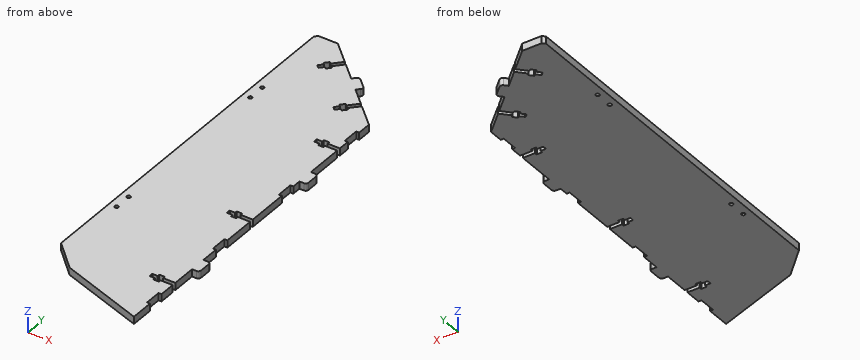
```python
from build123d import *

# Parameters (mm, degrees)
MODEL_R             = 1.6637
BOSS_EXTRUDE1_DEPTH = 6.6


with BuildPart() as part:
    # Model → Boss-Extrude1 (new body)
    with BuildSketch(Plane.XY):
        with BuildLine():
            Line((-2.7, 21.1), (0, 21.1))
            Line((0, 21.1), (0, 0))
            Line((0, 0), (-76.35, 26.1117))
            Line((-76.35, 26.1117), (-100, 49.2))
            Line((-100, 49.2), (-100, 380.9))
            Line((-100, 380.9), (-97.5, 383.4))
            Line((-97.5, 383.4), (-80, 383.4))
            Line((-80, 383.4), (-61.92031318, 366.450293606))
            Line((-61.92031318, 366.450293606), (-69.443665597, 358.42538436))
            Line((-69.443665597, 358.42538436), (-70.599982066, 359.50943105))
            ThreePointArc((-70.599982066, 359.50943105), (-70.958073277, 359.644402505), (-71.306721232, 359.486633012))
            Line((-71.306721232, 359.486633012), (-74.042485748, 356.568484196))
            ThreePointArc((-74.042485748, 356.568484196), (-74.177457203, 356.210392984), (-74.01968771, 355.861745029))
            Line((-74.01968771, 355.861745029), (-72.863371242, 354.77769834))
            Line((-72.863371242, 354.77769834), (-75.941106322, 351.494780921))
            ThreePointArc((-75.941106322, 351.494780921), (-76.076077777, 351.13668971), (-75.918308284, 350.788041755))
            Line((-75.918308284, 350.788041755), (-74.057988413, 349.043991876))
            ThreePointArc((-74.057988413, 349.043991876), (-73.699897202, 348.909020421), (-73.351249247, 349.066789913))
            Line((-73.351249247, 349.066789913), (-70.273514167, 352.349707332))
            Line((-70.273514167, 352.349707332), (-69.117197698, 351.265660643))
            ThreePointArc((-69.117197698, 351.265660643), (-68.759106487, 351.130689188), (-68.410458532, 351.288458681))
            Line((-68.410458532, 351.288458681), (-65.674694016, 354.206607497))
            ThreePointArc((-65.674694016, 354.206607497), (-65.539722561, 354.564698709), (-65.697492054, 354.913346664))
            Line((-65.697492054, 354.913346664), (-66.853808523, 355.997393353))
            Line((-66.853808523, 355.997393353), (-59.330456105, 364.022302598))
            Line((-59.330456105, 364.022302598), (-45.469249226, 351.02742115))
            Line((-45.469249226, 351.02742115), (-42.733484711, 353.945569966))
            ThreePointArc((-42.733484711, 353.945569966), (-40.990244935, 354.73441743), (-39.199788878, 354.059560154))
            Line((-39.199788878, 354.059560154), (-31.904416837, 347.220148866))
            ThreePointArc((-31.904416837, 347.220148866), (-31.115569373, 345.47690909), (-31.790426649, 343.686453033))
            Line((-31.790426649, 343.686453033), (-34.526191164, 340.768304216))
            Line((-34.526191164, 340.768304216), (-20.664984286, 327.773422768))
            Line((-20.664984286, 327.773422768), (-28.188336703, 319.748513522))
            Line((-28.188336703, 319.748513522), (-29.344653172, 320.832560211))
            ThreePointArc((-29.344653172, 320.832560211), (-29.702744383, 320.967531667), (-30.051392338, 320.809762174))
            Line((-30.051392338, 320.809762174), (-32.787156854, 317.891613357))
            ThreePointArc((-32.787156854, 317.891613357), (-32.922128309, 317.533522146), (-32.764358816, 317.184874191))
            Line((-32.764358816, 317.184874191), (-31.608042348, 316.100827502))
            Line((-31.608042348, 316.100827502), (-34.685777428, 312.817910083))
            ThreePointArc((-34.685777428, 312.817910083), (-34.820748883, 312.459818871), (-34.66297939, 312.111170916))
            Line((-34.66297939, 312.111170916), (-32.802659519, 310.367121038))
            ThreePointArc((-32.802659519, 310.367121038), (-32.444568308, 310.232149583), (-32.095920353, 310.389919075))
            Line((-32.095920353, 310.389919075), (-29.018185273, 313.672836494))
            Line((-29.018185273, 313.672836494), (-27.861868804, 312.588789805))
            ThreePointArc((-27.861868804, 312.588789805), (-27.503777593, 312.45381835), (-27.155129638, 312.611587842))
            Line((-27.155129638, 312.611587842), (-24.419365122, 315.529736659))
            ThreePointArc((-24.419365122, 315.529736659), (-24.284393667, 315.88782787), (-24.44216316, 316.236475825))
            Line((-24.44216316, 316.236475825), (-25.598479629, 317.320522515))
            Line((-25.598479629, 317.320522515), (-18.075127211, 325.34543176))
            Line((-18.075127211, 325.34543176), (0, 308.4))
            Line((0, 308.4), (0, 295.7))
            Line((0, 295.7), (-2.7, 295.7))
            Line((-2.7, 295.7), (-2.7, 280.7))
            Line((-2.7, 280.7), (0, 280.7))
            Line((0, 280.7), (0, 270.3))
            Line((0, 270.3), (-11, 270.3))
            Line((-11, 270.3), (-11, 271.885))
            ThreePointArc((-11, 271.885), (-11.146446609, 272.238553391), (-11.5, 272.385))
            Line((-11.5, 272.385), (-15.5, 272.385))
            ThreePointArc((-15.5, 272.385), (-15.853553391, 272.238553391), (-16, 271.885))
            Line((-16, 271.885), (-16, 270.3))
            Line((-16, 270.3), (-20.5, 270.3))
            ThreePointArc((-20.5, 270.3), (-20.853553391, 270.153553391), (-21, 269.8))
            Line((-21, 269.8), (-21, 267.25))
            ThreePointArc((-21, 267.25), (-20.853553391, 266.896446609), (-20.5, 266.75))
            Line((-20.5, 266.75), (-16, 266.75))
            Line((-16, 266.75), (-16, 265.165))
            ThreePointArc((-16, 265.165), (-15.853553391, 264.811446609), (-15.5, 264.665))
            Line((-15.5, 264.665), (-11.5, 264.665))
            ThreePointArc((-11.5, 264.665), (-11.146446609, 264.811446609), (-11, 265.165))
            Line((-11, 265.165), (-11, 266.75))
            Line((-11, 266.75), (0, 266.75))
            Line((0, 266.75), (0, 232.2))
            Line((0, 232.2), (4, 232.2))
            ThreePointArc((4, 232.2), (5.767766953, 231.467766953), (6.5, 229.7))
            Line((6.5, 229.7), (6.5, 219.7))
            ThreePointArc((6.5, 219.7), (5.767766953, 217.932233047), (4, 217.2))
            Line((4, 217.2), (0, 217.2))
            Line((0, 217.2), (0, 209.166666667))
            Line((0, 209.166666667), (-2.7, 209.166666667))
            Line((-2.7, 209.166666667), (-2.7, 194.166666667))
            Line((-2.7, 194.166666667), (0, 194.166666667))
            Line((0, 194.166666667), (0, 155.975))
            Line((0, 155.975), (-11, 155.975))
            Line((-11, 155.975), (-11, 157.56))
            ThreePointArc((-11, 157.56), (-11.146446609, 157.913553391), (-11.5, 158.06))
            Line((-11.5, 158.06), (-15.5, 158.06))
            ThreePointArc((-15.5, 158.06), (-15.853553391, 157.913553391), (-16, 157.56))
            Line((-16, 157.56), (-16, 155.975))
            Line((-16, 155.975), (-20.5, 155.975))
            ThreePointArc((-20.5, 155.975), (-20.853553391, 155.828553391), (-21, 155.475))
            Line((-21, 155.475), (-21, 152.925))
            ThreePointArc((-21, 152.925), (-20.853553391, 152.571446609), (-20.5, 152.425))
            Line((-20.5, 152.425), (-16, 152.425))
            Line((-16, 152.425), (-16, 150.84))
            ThreePointArc((-16, 150.84), (-15.853553391, 150.486446609), (-15.5, 150.34))
            Line((-15.5, 150.34), (-11.5, 150.34))
            ThreePointArc((-11.5, 150.34), (-11.146446609, 150.486446609), (-11, 150.84))
            Line((-11, 150.84), (-11, 152.425))
            Line((-11, 152.425), (0, 152.425))
            Line((0, 152.425), (0, 122.633333333))
            Line((0, 122.633333333), (-2.7, 122.633333333))
            Line((-2.7, 122.633333333), (-2.7, 107.633333333))
            Line((-2.7, 107.633333333), (0, 107.633333333))
            Line((0, 107.633333333), (0, 91.2))
            Line((0, 91.2), (4, 91.2))
            ThreePointArc((4, 91.2), (5.767766953, 90.467766953), (6.5, 88.7))
            Line((6.5, 88.7), (6.5, 78.7))
            ThreePointArc((6.5, 78.7), (5.767766953, 76.932233047), (4, 76.2))
            Line((4, 76.2), (0, 76.2))
            Line((0, 76.2), (0, 54.35))
            Line((0, 54.35), (-11, 54.35))
            Line((-11, 54.35), (-11, 55.935))
            ThreePointArc((-11, 55.935), (-11.146446609, 56.288553391), (-11.5, 56.435))
            Line((-11.5, 56.435), (-15.5, 56.435))
            ThreePointArc((-15.5, 56.435), (-15.853553391, 56.288553391), (-16, 55.935))
            Line((-16, 55.935), (-16, 54.35))
            Line((-16, 54.35), (-20.5, 54.35))
            ThreePointArc((-20.5, 54.35), (-20.853553391, 54.203553391), (-21, 53.85))
            Line((-21, 53.85), (-21, 51.3))
            ThreePointArc((-21, 51.3), (-20.853553391, 50.946446609), (-20.5, 50.8))
            Line((-20.5, 50.8), (-16, 50.8))
            Line((-16, 50.8), (-16, 49.215))
            ThreePointArc((-16, 49.215), (-15.853553391, 48.861446609), (-15.5, 48.715))
            Line((-15.5, 48.715), (-11.5, 48.715))
            ThreePointArc((-11.5, 48.715), (-11.146446609, 48.861446609), (-11, 49.215))
            Line((-11, 49.215), (-11, 50.8))
            Line((-11, 50.8), (0, 50.8))
            Line((0, 50.8), (0, 36.1))
            Line((0, 36.1), (-2.7, 36.1))
            Line((-2.7, 36.1), (-2.7, 21.1))
        make_face()
        with Locations((-93.2095625, 128.122348004)):
            Circle(MODEL_R, mode=Mode.SUBTRACT)
        with Locations((-93.2095625, 112.247348004)):
            Circle(MODEL_R, mode=Mode.SUBTRACT)
        with Locations((-93.2095625, 303.522348003)):
            Circle(MODEL_R, mode=Mode.SUBTRACT)
        with Locations((-93.2095625, 287.647348003)):
            Circle(MODEL_R, mode=Mode.SUBTRACT)
    extrude(amount=BOSS_EXTRUDE1_DEPTH)


solid = part.part
```
Work out the finished part from the listing and answer in its coordinate system (mm). Round coordinates to 2 decimals unless told otherwise and drop trailing zeros. Write each loop counter-clockwise with the first axis right and the second up, starting at its lowest first coordinate (ties: lowest second). Pieces come first, ordered by that corner, then holes.
1) A cutting plane is placed at C-C on y = 31.5. Determine the outline of the cut face in (x, z), and give its area (3 significant figures).
2) A cutting plane is placed at B-B on z = 5.5. Give the number of separate pieces and of enclosed holes in the cut face, and give its area (3 significant figures).
3) Consider probe 1 along Y at (x, z) = (-33, 5.75); probe 2 along X at (y, z) = (304, 4.5); probe 3 along X at (y, z) = (209.5, 1.5). Determine where each line is inside the solid, lowest interval first.
4) Flat-ended cylindrical pins translate along their axes: P1, Ø3.5, axis at y = 305, z = 3.5, coming from the +X side; P2, Ø2, axis at x = -17.5, z = 3, coming from the +Y side; P3, Ø2, axis at x = -54, z = 4, coming from the +Y side. Find the tip coordinate at first contact, or state that the pin passes through.
5) A cutting plane is placed at A-A on x = -51. Determine the outline of the cut face in (y, z).
Entries:
1. outline: (-81.87, 0) - (-2.7, 0) - (-2.7, 6.6) - (-81.87, 6.6) - close
1. area: 523 mm2
2. separate pieces: 1
2. enclosed holes: 4
2. area: 33,100 mm2
3. probe 1: y = 11.29 to 310.55, 314.62 to 339.34, 342.4 to 348.25
3. probe 2: x = -100 to -94.8, -91.62 to 0
3. probe 3: x = -100 to 0
4. P1: stops at x = 0
4. P2: stops at y = 325.35
4. P3: stops at y = 359.96
5. outline: (17.44, 0) - (356.21, 0) - (356.21, 6.6) - (17.44, 6.6) - close
